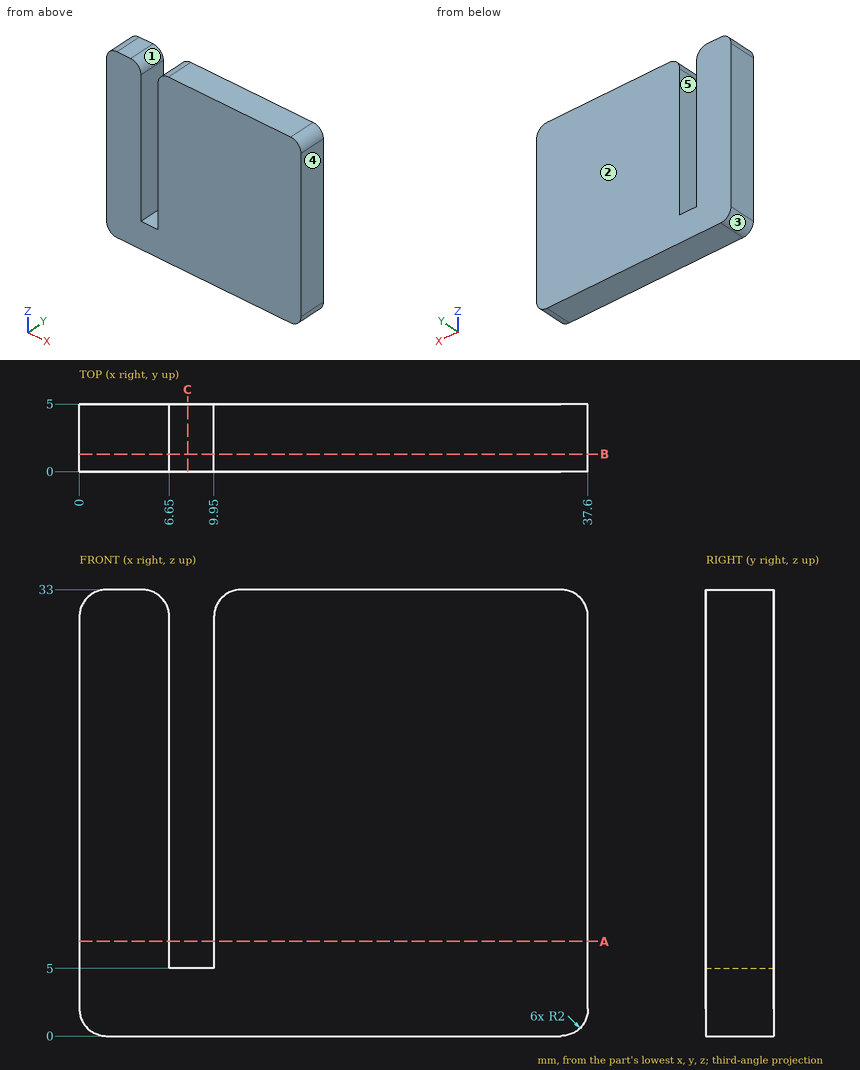
Verification items for this drawing (mm, ordinates from the low corner). A direction names the side the tool comes from. Coordinates: 2 decimals unless noted, no trailing zeros. Loops run counter-clockwise (first coordinate to the right, second up) from the corner with the lowest first, then second, coordinate; pieces in that order, holes last. Notation, with made-up numbers: (26.5, 70.25) - (85.5, 70.25) arc R19 ccw to (85.5, 98.25) - close; hole circle Ø7 at (68.5, 85). An arc over 180 degrees is marked (long way). One line per item, written item: value. Start each with the question number.
(1) Mould release check, pull along X, two halves, no side actions. Record for the marked faces 3, 4 and 5: released by +X, released by -X, zero draft, split by the parting line, or undercut.
(2) Cross-section at A-A on z = 7. Enter the section's corners in (x, y).
(3) Depth check by flat-ended pin: P1, Ø1.7, axis at x = 9, y = 3, coming from the +Z side. Enter the tip coordinate at first touch or a pass-through.
(4) Material ranges on line 1 (X direction, y = 1.3, z = 8); line 2 (Z direction, x = 7.5, y = 2.2), recorded low to high. Write a range as [from, to].
(5) Cross-section at B-B on y = 1.3. Enter the section's corners in (x, z).
(6) Tool access check on the marked faces 1 and 2. Record the directions out of +Z, -Z, +X, -X, +Y, -Y that give a thin tool (end or side, any length) a straight path to the whole face; none if there is none.
(7) Cross-section at C-C on x = 8. Enter the section's corners in (y, z), plus the area to 3 significant figures.
Results below:
1. face 3: released by -X
1. face 4: released by +X
1. face 5: undercut
2. outline: (0, 0) - (6.65, 0) - (6.65, 5) - (0, 5) - close; (9.95, 0) - (37.6, 0) - (37.6, 5) - (9.95, 5) - close
3. P1: stops at z = 5
4. line 1: x = [0, 6.65], [9.95, 37.6]
4. line 2: z = [0, 5]
5. outline: (0, 2) arc R2 ccw to (2, 0) - (35.6, 0) arc R2 ccw to (37.6, 2) - (37.6, 31) arc R2 ccw to (35.6, 33) - (11.95, 33) arc R2 ccw to (9.95, 31) - (9.95, 5) - (6.65, 5) - (6.65, 31) arc R2 ccw to (4.65, 33) - (2, 33) arc R2 ccw to (0, 31) - close
6. face 1: +Z, +Y, -Y
6. face 2: +Z, -Z, +X, -X, +Y
7. outline: (0, 0) - (5, 0) - (5, 5) - (0, 5) - close
7. area: 25.0 mm2
